from build123d import *

# Parameters (mm, degrees)
SKETCH1_W               = 15
SKETCH1_H               = 7.6
EXTRUDE1_DEPTH          = 10
SKETCH2_OUTSIDE_W       = 13.512
SKETCH2_OUTSIDE_H       = 15.912
CUT_EXTRUDE1_DEPTH      = 11
CUT_EXTRUDE1_DEPTH_BACK = 6
SKETCH3_R               = 1.65
SKETCH3_R_2             = 0.35
SKETCH3_W               = 0.4
SKETCH3_H               = 4
CUT_EXTRUDE2_DEPTH      = 4
SKETCH4_W               = 4
SKETCH4_H               = 5.5
CUT_EXTRUDE3_DEPTH      = 5.6
EXTRUDE3_DEPTH          = 6.5
CUT_EXTRUDE5_DEPTH      = 6.5
SKETCH10_W              = 1.1
SKETCH10_H              = 0.5
CUT_EXTRUDE6_DEPTH      = 3.6
SKETCH5_W               = 4
SKETCH5_H               = 5.1
EXTRUDE2_DEPTH          = 4.25
SKETCH6_R               = 1.6
CUT_EXTRUDE4_DEPTH      = 4.25
SKETCH11_R              = 0.5
EXTRUDE4_DEPTH          = 3.5
SKETCH12_R              = 1.65
EXTRUDE5_DEPTH          = 3
CUT_EXTRUDE7_DEPTH      = 0.4
EXTRUDE6_DEPTH          = 0.945
EXTRUDE9_DEPTH          = 0.39
LPATTERN1_COUNT         = 3
LPATTERN1_PITCH         = 5
FILLET1_R               = 0.3
FILLET2_R               = 0.7


with BuildPart() as part:
    # Sketch1 → Extrude1 (new body)
    with BuildSketch(Plane(origin=(0, 0, 0), x_dir=(1, 0, 0), z_dir=(0, 1, 0))):
        with Locations((2.5, 0)):
            Rectangle(SKETCH1_W, SKETCH1_H)
    extrude(amount=EXTRUDE1_DEPTH)

    # Sketch2 outside → Cut-Extrude1 (cut, two sides)
    with BuildSketch(Plane(origin=(0, 0, 0), x_dir=(0, 0, -1), z_dir=(1, 0, 0))) as cut_extrude1_sk:
        with Locations((0, 5)):
            Rectangle(SKETCH2_OUTSIDE_W, SKETCH2_OUTSIDE_H)
        Polygon((2.5, 10), (3.8, 6.5), (3.8, 0), (-3.8, 0), (-3.8, 6.5), (-2.5, 10), align=None, mode=Mode.SUBTRACT)
    extrude(amount=CUT_EXTRUDE1_DEPTH, mode=Mode.SUBTRACT)
    extrude(cut_extrude1_sk.sketch, amount=-CUT_EXTRUDE1_DEPTH_BACK, mode=Mode.SUBTRACT)

    # Sketch3 → Cut-Extrude2 (cut)
    with BuildSketch(Plane(origin=(0, 10, 0), x_dir=(-1, 0, 0), z_dir=(0, 1, 0))):
        with Locations((2.5, 0)):
            Circle(SKETCH3_R)
        with Locations((-2.5, 0)):
            Circle(SKETCH3_R)
        with Locations((2.5, -2.78)):
            Circle(SKETCH3_R_2)
        with Locations((-2.5, -2.78)):
            Circle(SKETCH3_R_2)
        with Locations((-7.5, 0)):
            Circle(SKETCH3_R)
        with Locations((-7.5, -2.78)):
            Circle(SKETCH3_R_2)
        Rectangle(SKETCH3_W, SKETCH3_H)
        with Locations((-5, 0)):
            Rectangle(SKETCH3_W, SKETCH3_H)
    extrude(amount=-CUT_EXTRUDE2_DEPTH, mode=Mode.SUBTRACT)

    # Sketch4 → Cut-Extrude3 (cut)
    with BuildSketch(Plane.XY.offset(3.8)):
        with Locations((-2.5, 3.25)):
            Rectangle(SKETCH4_W, SKETCH4_H)
        with Locations((2.5, 3.25)):
            Rectangle(SKETCH4_W, SKETCH4_H)
        with Locations((7.5, 3.25)):
            Rectangle(SKETCH4_W, SKETCH4_H)
    extrude(amount=-CUT_EXTRUDE3_DEPTH, mode=Mode.SUBTRACT)

    # Sketch7 → Extrude3 (add)
    with BuildSketch(Plane(origin=(0, 0, 0), x_dir=(1, 0, 0), z_dir=(0, 1, 0))):
        Polygon((-5.6, 3.1), (-5, 2.881617859), (-5, 2.118382141), (-5.6, 1.9), align=None)
    extrude(amount=EXTRUDE3_DEPTH)

    # Sketch9 → Cut-Extrude5 (cut)
    with BuildSketch(Plane(origin=(0, 0, 0), x_dir=(1, 0, 0), z_dir=(0, 1, 0))):
        Polygon((10, 2.881617859), (9.4, 3.1), (9.4, 1.9), (10, 2.118382141), align=None)
    extrude(amount=CUT_EXTRUDE5_DEPTH, mode=Mode.SUBTRACT)

    # Sketch10 → Cut-Extrude6 (cut)
    with BuildSketch(Plane.XY.offset(3.8)):
        with Locations((-2.5, 0.25)):
            Rectangle(SKETCH10_W, SKETCH10_H)
        with Locations((2.5, 0.25)):
            Rectangle(SKETCH10_W, SKETCH10_H)
        with Locations((7.5, 0.25)):
            Rectangle(SKETCH10_W, SKETCH10_H)
    extrude(amount=-CUT_EXTRUDE6_DEPTH, mode=Mode.SUBTRACT)

    # Sketch5 → Extrude2 (add)
    with BuildSketch(Plane.XY.offset(-1.8)):
        with Locations((-2.5, 3.05)):
            Rectangle(SKETCH5_W, SKETCH5_H)
        with Locations((2.5, 3.05)):
            Rectangle(SKETCH5_W, SKETCH5_H)
        with Locations((7.5, 3.05)):
            Rectangle(SKETCH5_W, SKETCH5_H)
    extrude(amount=EXTRUDE2_DEPTH)

    # Sketch6 → Cut-Extrude4 (cut)
    with BuildSketch(Plane.XY.offset(2.45)):
        with Locations((-2.5, 2.554263468)):
            Circle(SKETCH6_R)
        with Locations((2.5, 2.554263468)):
            Circle(SKETCH6_R)
        with Locations((7.5, 2.554263468)):
            Circle(SKETCH6_R)
    extrude(amount=-CUT_EXTRUDE4_DEPTH, mode=Mode.SUBTRACT)

    # Sketch11 → Extrude4 (add)
    with BuildSketch(Plane.XZ.offset(-0.5)):
        with Locations((-2.5, 0.8)):
            Circle(SKETCH11_R)
        with Locations((2.5, 0.8)):
            Circle(SKETCH11_R)
        with Locations((7.5, 0.8)):
            Circle(SKETCH11_R)
    extrude(amount=EXTRUDE4_DEPTH)

    # Sketch12 → Extrude5 (add)
    with BuildSketch(Plane.XZ.offset(-6)):
        with Locations((2.5, 0)):
            Circle(SKETCH12_R)
        with Locations((-2.5, 0)):
            Circle(SKETCH12_R)
        with Locations((7.5, 0)):
            Circle(SKETCH12_R)
    extrude(amount=-EXTRUDE5_DEPTH)

    # Sketch13 → Cut-Extrude7 (cut)
    with BuildSketch(Plane(origin=(0, 9, 0), x_dir=(-1, 0, 0), z_dir=(0, 1, 0))):
        with BuildLine():
            Line((3.594307251, -1.234905519), (1.825829895, 1.505986278))
            ThreePointArc((1.825829895, 1.505986278), (1.605433494, 1.386452583), (1.405692749, 1.234905519))
            Line((1.405692749, 1.234905519), (3.174170105, -1.505986278))
            ThreePointArc((3.174170105, -1.505986278), (3.394566506, -1.386452583), (3.594307251, -1.234905519))
        make_face()
        with BuildLine():
            Line((-5.938894906, -0.534276038), (-9.149461674, 0.042144841))
            ThreePointArc((-9.149461674, 0.042144841), (-9.12403295, 0.291576712), (-9.061105094, 0.534276038))
            Line((-9.061105094, 0.534276038), (-5.850538326, -0.042144841))
            ThreePointArc((-5.850538326, -0.042144841), (-5.87596705, -0.291576712), (-5.938894906, -0.534276038))
        make_face()
        with BuildLine():
            Line((-2.83217089, -1.616218581), (-1.698971441, 1.44251629))
            ThreePointArc((-1.698971441, 1.44251629), (-1.926782442, 1.54723031), (-2.16782911, 1.616218581))
            Line((-2.16782911, 1.616218581), (-3.301028559, -1.44251629))
            ThreePointArc((-3.301028559, -1.44251629), (-3.073217558, -1.54723031), (-2.83217089, -1.616218581))
        make_face()
    extrude(amount=-CUT_EXTRUDE7_DEPTH, mode=Mode.SUBTRACT)

    # Sketch14 → Extrude6 (add, symmetric)
    with BuildSketch(Plane.ZY.offset(2.5)):
        Polygon((2.45, 5.6), (3.03887637, 3.861674443), (0.167170254, 1.787608865), (-0.546359637, 2.097431054), (-0.705673534, 1.730526322), (0.216750724, 1.33), (3.512480259, 3.710312924), (2.736824279, 6), (-1.8, 6), (-1.8, 5.6), align=None)
    extrude6 = extrude(amount=EXTRUDE6_DEPTH, both=True)

    # Sketch15 → Extrude9 (add)
    with BuildSketch(Plane(origin=(0, 1.449355072, 4.278403908), x_dir=(1, 0, 0), z_dir=(0, 0.320850379, 0.947129893))):
        Polygon((-1.555, 4.8), (-1.555, 2.903968921), (-0.51, 4.8), align=None)
        Polygon((-3.445, 4.8), (-3.445, 2.903968921), (-4.49, 4.8), align=None)
    extrude9 = extrude(amount=-EXTRUDE9_DEPTH)

    # LPattern1: Extrude6, Extrude9 ×3
    with Locations(*[(i * LPATTERN1_PITCH, 0, 0) for i in range(1, LPATTERN1_COUNT)]):
        add(extrude6)
        add(extrude9)

    # Fillet1
    fillet1_edges = [part.edges().sort_by_distance(p)[0] for p in [
        (-2.5, 3.861674443, 3.03887637),
        (-2.5, 1.787608865, 0.167170254),
        (2.5, 3.861674443, 3.03887637),
        (2.5, 1.787608865, 0.167170254),
        (7.5, 3.861674443, 3.03887637),
        (7.5, 1.787608865, 0.167170254),
    ]]
    fillet(fillet1_edges, radius=FILLET1_R)

    # Fillet2
    fillet2_edges = [part.edges().sort_by_distance(p)[0] for p in [
        (-2.5, 3.710312924, 3.512480259),
        (-2.5, 1.33, 0.216750724),
        (2.5, 1.33, 0.216750724),
        (2.5, 3.710312924, 3.512480259),
        (7.5, 3.710312924, 3.512480259),
        (7.5, 1.33, 0.216750724),
    ]]
    fillet(fillet2_edges, radius=FILLET2_R)


solid = part.part
Could you check a few things on this model? Use its own coordinates, in mm. A direction names the side the tool comes from. Coordinates: 2 decimals unless noted, no trailing zeros. Order: outer loops, then holes, each group sorted by start corner. A loop starts at its lowest first (then second) coordinate and runs counter-clockwise, first axis right, second up. Notation, with made-up numbers: (63, -5.5) - (122, -5.5) arc R11 ccw to (122, -0.5) - close; hole circle Ø5 at (17, 84.5). An arc over 180 degrees is marked (long way). Answer in a Markdown table with one row per item. Add a question column.
(1) I need wall thicknesses on L1, parallel to Y at x = 6.5, z = 0.5; L2, parallel to X at y = 9.4, z = 0; L3, parallel to Y at x = 6.5, z = 0. Which ranges of each line are inside material? Lowest first, please.
(2) If we section it at C-C, the plane z = 0.8: State how many separate pieces and enclosed holes the cut face has, then the cut area to 3 significant figures.
(3) Will these pins go through, and if not, where does the flat tip stop? pin 1 (0.5 mm diameter, centred on x = 6, z = -0.5, fed in from +Y); pin 2 (0.7 mm diameter, centred on x = -2, z = 0, fed in from +Y); pin 3 (2.5 mm diameter, centred on y = 5, z = 1, fed in from -X).
(4) If we mould it in two halves opening along Z, with no side actions, what happens to faces 5 (the face through (-4, 0.5, 3)), 6 (the face through (-2.513, 2.473, 1.799)), 7 (the face through (4, 5.6, 0))? For each: released by +Z, released by -Z, zero draft, split by the parting line, or undercut.
(5) If we section it at A-A, the plane x = 8.75: Please give me the cut outline in (y, z), then the cut area to 3 significant figures.
(6) On a 3-axis mill with a long thin cutter (end or side, diameter ignored), from which of +Z, -Z, +X, -X, +Y, -Y can I reach the whole of each face in a straight line? I mean faces 1 (the face through (1, 5.6, 0)), 2 (the face through (7.487, 2.473, 1.799)), 3 (the face through (10, 5, 0)), 4 (the face through (-0.2, 8, 0)). Say none if no direction works.
(7) If we section it at B-B, the plane x = 0: Please give me the cut outline in (y, z), then the cut area to 4 significant figures.
Results are:
| question | item | result |
|---|---|---|
| 1 | L1 | y = 0 to 1.31, 3.8 to 5.6, 6 to 9 |
| 1 | L2 | x = -5 to -4.15, -0.85 to -0.2, 0.2 to 0.85, 4.15 to 4.8, 5.2 to 5.85, 9.15 to 10 |
| 1 | L3 | y = 0 to 1.31, 3.8 to 5.6, 6 to 8.6 |
| 2 | separate pieces | 4 |
| 2 | enclosed holes | 9 |
| 2 | area | 123 mm2 |
| 3 | pin 1 | stops at y = 10 |
| 3 | pin 2 | stops at y = 9 |
| 3 | pin 3 | stops at x = -5 |
| 4 | face 5 | zero draft |
| 4 | face 6 | released by +Z |
| 4 | face 7 | undercut |
| 5 | outline | (0, -3.8) - (6.5, -3.8) - (10, -2.5) - (10, -1.08) - (9, -1.08) - (9, -0.03) - (8.6, -0.03) - (8.6, 0.48) - (9, 0.48) - (9, 1.08) - (10, 1.08) - (10, 2.5) - (6.5, 3.8) - (6, 3.8) - (6, -1.8) - (5.6, -1.8) - (5.6, 2.45) - (3.55, 2.45) - (3.55, -1.8) - (1.56, -1.8) - (1.56, 2.45) - (0.5, 2.45) - (0.5, 3.8) - (0, 3.8) - close; (4.6, 2.8) - (5.87, 2.37) - (6, 2.74) - (4.72, 3.17) - close |
| 5 | area | 52.0 mm2 |
| 6 | face 1 | none |
| 6 | face 2 | +Z |
| 6 | face 3 | +Z, -Z, +X, +Y, -Y |
| 6 | face 4 | +Y |
| 7 | outline | (0, -3.8) - (6.5, -3.8) - (10, -2.5) - (10, -2) - (6, -2) - (6, 2) - (10, 2) - (10, 2.5) - (6.5, 3.8) - (0, 3.8) - close |
| 7 | area | 55.45 mm2 |
